```python
from build123d import *

# Parameters (mm, degrees)
BOSS_EXTRUDE1_DEPTH      = 5.1
BOSS_EXTRUDE1_DEPTH_BACK = 5.1
SKETCH1_R                = 1.55
BOSS_EXTRUDE2_DEPTH      = 5.15
BOSS_EXTRUDE2_DEPTH_BACK = 5.15
SKETCH1_3_R              = 1.55
BOSS_EXTRUDE3_DEPTH      = 2.4
BOSS_EXTRUDE3_DEPTH_BACK = 2.4
SKETCH1_4_R              = 2.4
SKETCH1_4_W              = 10
SKETCH1_4_H              = 0.5


with BuildPart() as part:
    # Sketch1 → Boss-Extrude1 (new, two sides: drawn at the far end of the back side and taken through both)
    with BuildSketch(Plane.XY.offset(-BOSS_EXTRUDE1_DEPTH_BACK)):
        with BuildLine():
            Line((5.8, 2.8), (5.8, 0))
            Line((5.8, 0), (15.802181202, 0))
            Line((15.802181202, 0), (16.302181202, 0))
            Line((16.302181202, 0), (24.8, 0))
            ThreePointArc((24.8, 0), (26.921320344, 0.878679656), (27.8, 3))
            Line((27.8, 3), (27.8, 5.8))
            Line((27.8, 5.8), (27.8, 6.3))
            Line((27.8, 6.3), (27.8, 9.6))
            Line((27.8, 9.6), (27.8, 10.1))
            Line((27.8, 10.1), (25, 10.1))
            ThreePointArc((25, 10.1), (22.878679656, 10.978679656), (22, 13.1))
            Line((22, 13.1), (22, 15.9))
            Line((22, 15.9), (16.9, 15.9))
            Line((16.9, 15.9), (16.4, 15.9))
            Line((16.4, 15.9), (5.8, 15.9))
            Line((5.8, 15.9), (4.5, 15.9))
            Line((4.5, 15.9), (3, 15.9))
            ThreePointArc((3, 15.9), (0.878679656, 15.021320344), (0, 12.9))
            Line((0, 12.9), (0, 5.8))
            Line((0, 5.8), (2.8, 5.8))
            ThreePointArc((2.8, 5.8), (4.921320344, 4.921320344), (5.8, 2.8))
        make_face()
        with Locations((13.9, 13.1)):
            Circle(SKETCH1_R, mode=Mode.SUBTRACT)
    extrude(amount=BOSS_EXTRUDE1_DEPTH + BOSS_EXTRUDE1_DEPTH_BACK)

    # Sketch1_3 → Boss-Extrude2 (add, two sides: drawn at the far end of the back side and taken through both)
    # profile 1 of 2: a face of its own
    with BuildSketch(Plane.XY.offset(-BOSS_EXTRUDE2_DEPTH_BACK)):
        with BuildLine():
            ThreePointArc((0, 3), (0.878679656, 0.878679656), (3, 0))
            Line((3, 0), (5.8, 0))
            Line((5.8, 0), (5.8, 2.8))
            ThreePointArc((5.8, 2.8), (4.921320344, 4.921320344), (2.8, 5.8))
            Line((2.8, 5.8), (0, 5.8))
            Line((0, 5.8), (0, 3))
        make_face()
        with BuildLine():
            Line((3.498212002, 1.25), (2.101787998, 1.25))
            ThreePointArc((2.101787998, 1.25), (1.1, 2.8), (2.101787998, 4.35))
            Line((2.101787998, 4.35), (3.498212002, 4.35))
            ThreePointArc((3.498212002, 4.35), (4.5, 2.8), (3.498212002, 1.25))
        make_face(mode=Mode.SUBTRACT)
    # profile 2 of 2: a face of its own
    with BuildSketch(Plane.XY.offset(-BOSS_EXTRUDE2_DEPTH_BACK)):
        with BuildLine():
            Line((25, 10.1), (27.8, 10.1))
            Line((27.8, 10.1), (27.8, 12.9))
            ThreePointArc((27.8, 12.9), (26.921320344, 15.021320344), (24.8, 15.9))
            Line((24.8, 15.9), (22, 15.9))
            Line((22, 15.9), (22, 13.1))
            ThreePointArc((22, 13.1), (22.878679656, 10.978679656), (25, 10.1))
        make_face()
        with Locations((25, 13.1)):
            Circle(SKETCH1_3_R, mode=Mode.SUBTRACT)
    extrude(amount=BOSS_EXTRUDE2_DEPTH + BOSS_EXTRUDE2_DEPTH_BACK)

    # Sketch1_4 → Boss-Extrude3 (add, two sides: drawn at the far end of the back side and taken through both)
    with BuildSketch(Plane.XY.offset(-BOSS_EXTRUDE3_DEPTH_BACK)):
        with Locations((-9, 21.1)):
            Circle(SKETCH1_4_R)
        Polygon((16.4, 17.9), (16.4, 15.9), (16.9, 15.9), (16.9, 18.4), (-6.6, 18.4), (-6.6, 17.9), (5, 17.9), (5.3, 17.9), align=None)
        with BuildLine():
            Line((4.5, 17.4), (4.5, 15.9))
            Line((4.5, 15.9), (5.8, 15.9))
            Line((5.8, 15.9), (5.8, 17.4))
            ThreePointArc((5.8, 17.4), (5.653553391, 17.753553391), (5.3, 17.9))
            Line((5.3, 17.9), (5, 17.9))
            ThreePointArc((5, 17.9), (4.646446609, 17.753553391), (4.5, 17.4))
        make_face()
        with Locations((32.8, 6.05)):
            Rectangle(SKETCH1_4_W, SKETCH1_4_H)
        with Locations((32.8, 9.85)):
            Rectangle(SKETCH1_4_W, SKETCH1_4_H)
        with BuildLine():
            Line((16.302181202, 0), (15.802181202, 0))
            Line((15.802181202, 0), (15.802181202, -2.4))
            ThreePointArc((15.802181202, -2.4), (15.948627812, -2.753553391), (16.302181202, -2.9))
            Line((16.302181202, -2.9), (24.80383619, -2.9))
            Line((24.80383619, -2.9), (24.80383619, -2.4))
            Line((24.80383619, -2.4), (16.302181202, -2.4))
            Line((16.302181202, -2.4), (16.302181202, 0))
        make_face()
        with BuildLine():
            Line((-11.4, 17.9), (-6.6, 17.9))
            Line((-6.6, 17.9), (-6.6, 18.4))
            Line((-6.6, 18.4), (-6.6, 21.1))
            ThreePointArc((-6.6, 21.1), (-9, 18.7), (-11.4, 21.1))
            Line((-11.4, 21.1), (-11.4, 17.9))
        make_face()
    extrude(amount=BOSS_EXTRUDE3_DEPTH + BOSS_EXTRUDE3_DEPTH_BACK)


solid = part.part
```
Here's how the part is built. I have some questions about the finished solid (model axes, mm). A direction names the side the tool comes from. Round coordinates to 2 decimals unless told otherwise and drop trailing zeros. Order: outer loops, then holes, each group sorted by start corner. A loop starts at its lowest first (then second) coordinate and runs counter-clockwise, first axis right, second up. Notation, with made-up numbers: M 44,61 L 65,61 A12 ccw 65,73 Z; hole C 56.25,-17.5 d7. An arc over 180 degrees is marked long. Use CSV: the item, a comma, the result in double quotes.
1) On a 3-axis mill with a long thin cutter (end or side, diameter ignored), from which of +Z, -Z, +X, -X, +Y, -Y can I reach the whole of each face in a straight line? I mean faces 4 (the flat face through (33, 5.8, 0)), 5 (the cylindrical face through (0.9, 15.04, -0.07)), 6 (the flat face through (19.3, -2.6, 2.4)), 7 (the cylindrical face through (4.5, 2.8, -0.1)). Say none if no direction works.
Taken from the geometry:
face 4,"+Z, -Z, +X, -Y"
face 5,"+Z, -Z, -X"
face 6,"+Z, +X, -X, -Y"
face 7,"+Z, -Z"
2) If we mould it in two halves opening along X, with no side actions, what happens to faces 1 (the flat face through (11, 17.9, 0)), 2 (the cylindrical face through (0.86, 0.9, -0.07)), 3 (the flat face through (5, 18.4, 0))? For each: pulls with the +X half, pulls with the -X half, needs draft (parallel to the pull), parting line crosses it, or undercut.
Taken from the geometry:
face 1,"undercut"
face 2,"pulls with the -X half"
face 3,"needs draft"
3) I want a section at B-B (x = 13.9). List the corners of the cut face in (y, z) for me, then the cut area to 3 significant figures.
Taken from the geometry:
outline,"M 0,-5.1 L 11.55,-5.1 L 11.55,5.1 L 0,5.1 Z; M 14.65,-5.1 L 15.9,-5.1 L 15.9,5.1 L 14.65,5.1 Z; M 17.9,-2.4 L 18.4,-2.4 L 18.4,2.4 L 17.9,2.4 Z"
area,"133 mm^2"
4) I want a section at D-D (y = 8.5). List the corners of the cut face in (x, z) for me.
Taken from the geometry:
outline,"M 0,-5.1 L 27.8,-5.1 L 27.8,5.1 L 0,5.1 Z"
5) I want a section at A-A (x = 8.5). List the corners of the cut face in (y, z) for me, then the cut area to 3 significant figures.
Taken from the geometry:
outline,"M 0,-5.1 L 15.9,-5.1 L 15.9,5.1 L 0,5.1 Z; M 17.9,-2.4 L 18.4,-2.4 L 18.4,2.4 L 17.9,2.4 Z"
area,"165 mm^2"
6) I want a section at C-C (z = 1.5). Count the separate pieces of the cut face and the enclosed holes in it, then the cut area to 3 significant figures.
Taken from the geometry:
separate pieces,"1"
enclosed holes,"4"
area,"466 mm^2"
7) I need wall thicknesses on line 1 along Y through (x, z) = (13.9, -2); line 2 along Y through (x, z) = (13.9, -2.5); line 3 along X through (y, z) = (12.25, 1). Which ranges of each line are inside material? Lowest first, please. Write a range as [from, to].
Taken from the geometry:
line 1,"[0, 11.55], [14.65, 15.9], [17.9, 18.4]"
line 2,"[0, 11.55], [14.65, 15.9]"
line 3,"[0, 12.6], [15.2, 23.7], [26.3, 27.8]"
8) I'm going to push flat-ended pins straight in: P1, Ø1, axis at x = -5.5, y = 16.5, coming from the +Z side; P2, Ø1.6, axis at y = 17, z = 0, coming from the -X side; P3, Ø1.4, axis at x = 34.5, z = 1, coming from the -Y side; P4, Ø4, axis at x = -1.5, z = 0.5, coming from the -Y side. Where does each tip first touch, or does it pass through?
Taken from the geometry:
P1,"through"
P2,"x = 4.5"
P3,"y = 5.8"
P4,"y = 1.34"
